Job drawing, mm, ordinate dimensions from the low corner. One solid piece. A direction names the side the tool comes from. Round coordinates to 2 decimals unless told otherwise and drop trailing zeros. Write each loop counter-clockwise with the first axis right and the second up, starting at its lowest first coordinate (ties: lowest second). Pieces come first, ordered by that corner, then holes.
1) Saw through at B-B on y = 7.75. Write the cut outline in (x, z), and give its area (3 significant figures).
2) Saw through at A-A on z = 2.5. Write the cut outline in (x, y), and give its area (3 significant figures).
3) Which spindle directions (+Z, -Z, +X, -X, +Y, -Y) get a long thin tool onto all of the face, cutting with end or side? Do the marked faces 1, 2 and 3. Say none if no direction does.
4) Saw through at D-D on z = 4.05. Write the cut outline in (x, y).
5) Flat gauge pins, fed straight in: pin 1 (1.1 mm diameter, centred on x = 4.5, z = 3, fed in from +Y); pin 2 (2 mm diameter, centred on y = 9.5, z = 2, fed in from +X); pin 3 (2 mm diameter, centred on y = 10, z = 3, fed in from -X); pin 4 (0.8 mm diameter, centred on x = 0.5, z = 3.5, fed in from +Y). Where does each tip first touch, or does it go through?
6) Saw through at C-C on x = 1.2. Write the cut outline in (y, z), and give its area (3 significant figures).
7) Drill centre lines: L1, parallel to X at y = 9.5, z = 2.1; L2, parallel to Y at x = 4.1, z = 3.35; L3, parallel to Z at x = 2.3, y = 11.5. Where is each one in solid material? Low to high.
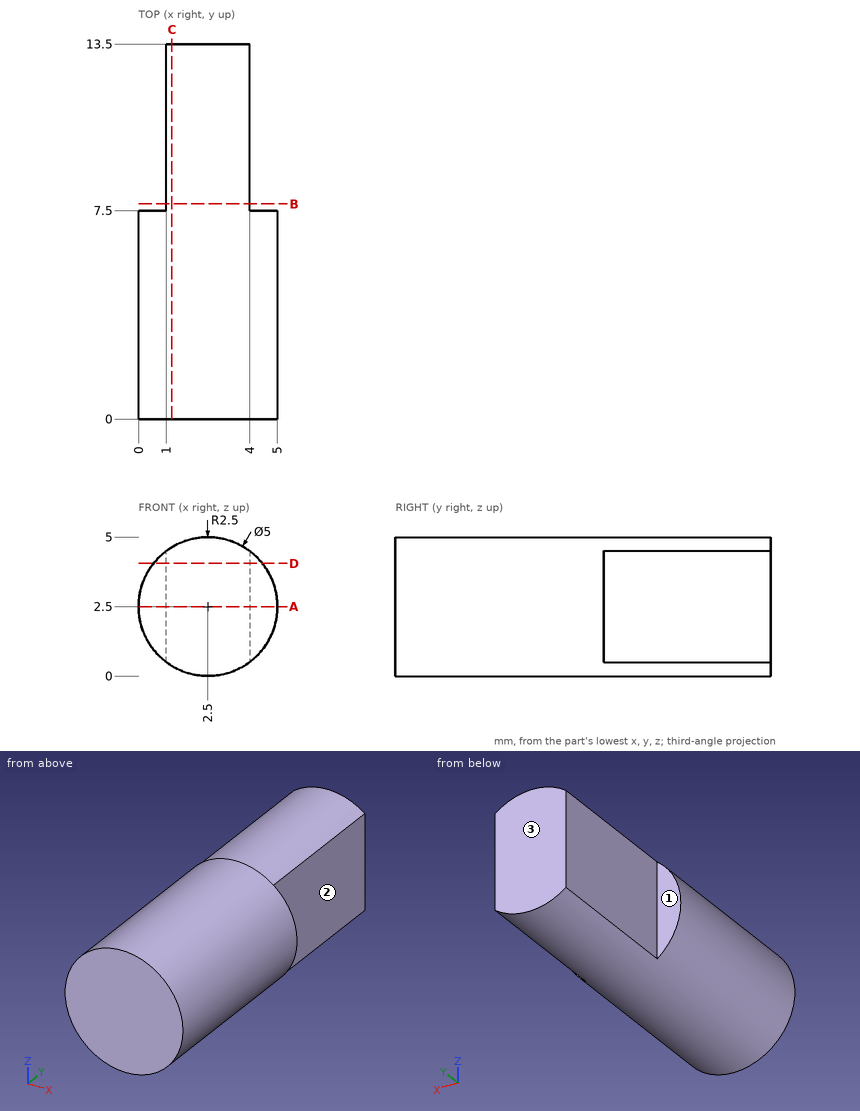
Completed:
1. outline: (1, 0.5) arc R2.5 ccw to (4, 0.5) - (4, 4.5) arc R2.5 ccw to (1, 4.5) - close
1. area: 14.0 mm2
2. outline: (0, 0) - (5, 0) - (5, 7.5) - (4, 7.5) - (4, 13.5) - (1, 13.5) - (1, 7.5) - (0, 7.5) - close
2. area: 55.5 mm2
3. face 1: +Z, -Z, -X, +Y
3. face 2: +Z, -Z, +X, +Y
3. face 3: +Z, -Z, +X, -X, +Y
4. outline: (0.54, 0) - (4.46, 0) - (4.46, 7.5) - (4, 7.5) - (4, 13.5) - (1, 13.5) - (1, 7.5) - (0.54, 7.5) - close
5. pin 1: stops at y = 13.5
5. pin 2: stops at x = 4
5. pin 3: stops at x = 1
5. pin 4: stops at y = 7.5
6. outline: (0, 0.36) - (13.5, 0.36) - (13.5, 4.64) - (0, 4.64) - close
6. area: 57.7 mm2
7. L1: x = 1 to 4
7. L2: y = 0 to 7.5
7. L3: z = 0.01 to 4.99
